from build123d import *

# Parameters (mm, degrees)
EXTRUDE_1_DEPTH     = 105
SKETCH_2_R          = 1.65
CUT_EXTRUDE_1_DEPTH = 107.056777247


with BuildPart() as part:
    # 草图1 → 凸台-拉伸1 (new body)
    with BuildSketch(Plane(origin=(0, 0, 0), x_dir=(1, 0, 0), z_dir=(0, 1, 0))):
        Polygon((0, 0), (0, 1.4), (1, 1.4), (1, 2.9), (0, 2.9), (0, 5.2), (14, 5.2), (14, 2.9), (13, 2.9), (13, 1.4), (14, 1.4), (14, 0), align=None)
    extrude(amount=EXTRUDE_1_DEPTH)

    # 草图2 → 切除-拉伸1 (cut, through all)
    with BuildSketch(Plane(origin=(0, 0, -5.2), x_dir=(-1, 0, 0), z_dir=(0, 0, -1))):
        with Locations((-7, 52.5)):
            Circle(SKETCH_2_R)
        with Locations((-7, 82.5)):
            Circle(SKETCH_2_R)
        with Locations((-7, 22.5)):
            Circle(SKETCH_2_R)
    extrude(amount=-CUT_EXTRUDE_1_DEPTH, mode=Mode.SUBTRACT)


solid = part.part
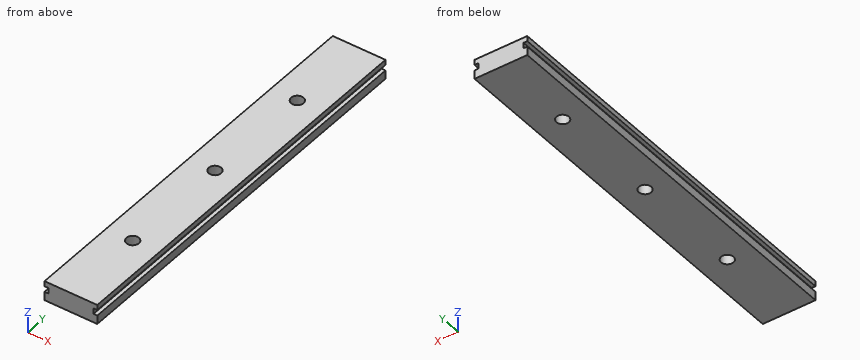
Verification items for the finished model (mm, model axes). Coordinates: 2 decimals unless noted, no trailing zeros. Write each loop counter-clockwise with the first axis right and the second up, starting at its lowest first coordinate (ties: lowest second). Pieces come first, ordered by that corner, then holes. Notation, with made-up numbers: (84.25, -18.75) -> (118.25, -18.75) arc R21 ccw to (118.25, 4.25) -> close; hole circle Ø3 at (-27, 68). An arc over 180 degrees is marked (long way). One line per item, written item: value. Start each with the question number.
Q1. Cross-section at B-B on x = 7. Enter the section's corners in (y, z), and give its area (3 significant figures).
Q2. Go/stop test with a flat-tipped pin: P1, Ø3, axis at x = 7, y = 22.5, coming from the -Z side (1 decimal). Record where the tip stops, or that it passes through.
Q3. Thickness scan on L1, parallel to Y at x = 7.25, z = -1.7; L2, parallel to Y at x = 8.5, z = -0.2; L3, parallel to X at y = 82.5, z = -2.4. Record the ranges inside material, lowest first. Write a range as from..to.
Q4. Cross-section at C-C on y = 36. Enter the section's corners in (x, z).
Q5. Cross-section at A-A on y = 82.5. Enter the section's corners in (x, z).
Checked values:
1. outline: (0, -5.2) -> (20.85, -5.2) -> (20.85, 0) -> (0, 0) -> close; (24.15, -5.2) -> (50.85, -5.2) -> (50.85, 0) -> (24.15, 0) -> close; (54.15, -5.2) -> (80.85, -5.2) -> (80.85, 0) -> (54.15, 0) -> close; (84.15, -5.2) -> (105, -5.2) -> (105, 0) -> (84.15, 0) -> close
1. area: 495 mm²
2. P1: passes through
3. L1: y = 0..20.87, 24.13..50.87, 54.13..80.87, 84.13..105
3. L2: y = 0..21.81, 23.19..51.81, 53.19..81.81, 83.19..105
3. L3: x = 1..5.35, 8.65..13
4. outline: (0, -5.2) -> (14, -5.2) -> (14, -2.9) -> (13, -2.9) -> (13, -1.4) -> (14, -1.4) -> (14, 0) -> (0, 0) -> (0, -1.4) -> (1, -1.4) -> (1, -2.9) -> (0, -2.9) -> close
5. outline: (0, -5.2) -> (5.35, -5.2) -> (5.35, 0) -> (0, 0) -> (0, -1.4) -> (1, -1.4) -> (1, -2.9) -> (0, -2.9) -> close; (8.65, -5.2) -> (14, -5.2) -> (14, -2.9) -> (13, -2.9) -> (13, -1.4) -> (14, -1.4) -> (14, 0) -> (8.65, 0) -> close
